Read the model definition and answer for the solid it produces. Units are mm, in the model's axes. Face numbers are marked on the shaded views. A direction names the side the tool comes from. Coordinates: 2 decimals unless noted, no trailing zeros. Order: outer loops, then holes, each group sorted by start corner. A loop starts at its lowest first (then second) coordinate and runs counter-clockwise, first axis right, second up. Notation, with made-up numbers: (-8.75, 72) -> (30.25, 72) arc R31 ccw to (30.25, 97) -> close; hole circle Ø6 at (-12.75, 50). An arc over 180 degrees is marked (long way). Return JSON: item names as keys, results as strings. Group by question number.
```python
from build123d import *

# Parameters (mm, degrees)
CASE_23X12P2X23_START                = -19
CASE_23X12P2X23_PROFILE_W            = 23
CASE_23X12P2X23_PROFILE_H            = 12.2
CASE_23X12P2X23_DEPTH                = 23
MOUNTING_EARS_33X12P2_START          = -2
MOUNTING_EARS_33X12P2_PROFILE_W      = 33
MOUNTING_EARS_33X12P2_PROFILE_H      = 12.2
MOUNTING_EARS_33X12P2_DEPTH          = 2
OUTPUT_ENVELOPE_NOT_SPLINE_START     = 4
OUTPUT_ENVELOPE_NOT_SPLINE_PROFILE_R = 2.5
OUTPUT_ENVELOPE_NOT_SPLINE_DEPTH     = 5
MOUNTING_HOLES_NOMINAL_START         = -50
MOUNTING_HOLES_NOMINAL_PROFILE_R     = 1.1
MOUNTING_HOLES_NOMINAL_DEPTH         = 80.702020133


with BuildPart() as part:
    # Case_23x12p2x23_profile → Case_23x12p2x23 (new body)
    with BuildSketch(Plane.XY.offset(CASE_23X12P2X23_START)):
        with Locations((5.5, 0)):
            Rectangle(CASE_23X12P2X23_PROFILE_W, CASE_23X12P2X23_PROFILE_H)
    extrude(amount=CASE_23X12P2X23_DEPTH)

    # Mounting_ears_33x12p2_profile → Mounting_ears_33x12p2 (add)
    with BuildSketch(Plane.XY.offset(MOUNTING_EARS_33X12P2_START)):
        with Locations((5.5, 0)):
            Rectangle(MOUNTING_EARS_33X12P2_PROFILE_W, MOUNTING_EARS_33X12P2_PROFILE_H)
    extrude(amount=MOUNTING_EARS_33X12P2_DEPTH)

    # Output_envelope_not_spline_profile → Output_envelope_not_spline (add)
    with BuildSketch(Plane.XY.offset(OUTPUT_ENVELOPE_NOT_SPLINE_START)):
        Circle(OUTPUT_ENVELOPE_NOT_SPLINE_PROFILE_R)
    extrude(amount=OUTPUT_ENVELOPE_NOT_SPLINE_DEPTH)

    # Mounting_holes_nominal_profile → Mounting_holes_nominal (cut, through all)
    with BuildSketch(Plane.XY.offset(MOUNTING_HOLES_NOMINAL_START)):
        with Locations(Location((-9, 0, 0), (0, 0, 180))):
            Circle(MOUNTING_HOLES_NOMINAL_PROFILE_R)
        with Locations(Location((20, 0, 0), (0, 0, 180))):
            Circle(MOUNTING_HOLES_NOMINAL_PROFILE_R)
    extrude(amount=MOUNTING_HOLES_NOMINAL_DEPTH, mode=Mode.SUBTRACT)


solid = part.part
```
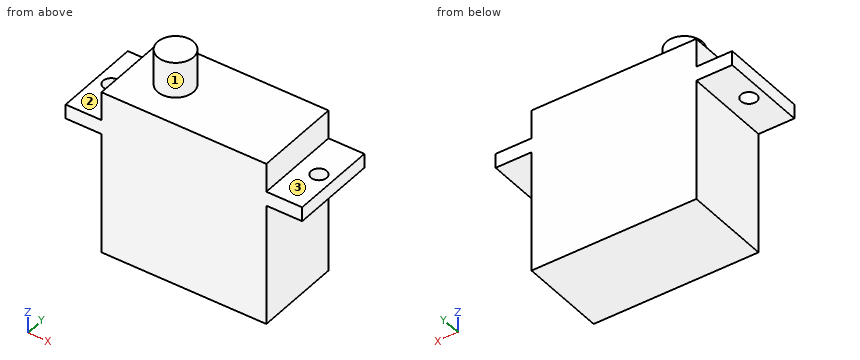
1. Straight lines are drawn through the part: L1, parallel to Y at x = -9, z = -1.4; L2, parallel to X at y = 2.75, z = -10.25; L3, parallel to Z at x = 20.5, y = -1.75. For each, find the intervals that lie inside material, in ascending order.
2. Find section A-A on x = -9. Determine the outline of the cut face in (y, z), and give its area (3 significant figures).
3. Find section D-D on y = 2. Determine the outline of the cut face in (x, z).
4. Find section C-C on x = 0. Determine the outline of the cut face in (y, z), and give its area (3 significant figures).
5. Given pin 1 (1.5 mm diameter, centred on y = -4, z = -9.5, fed in from +X); pin 2 (2 mm diameter, centred on y = -0.5, z = 3, fed in from -X); pin 3 (2.5 mm diameter, centred on x = -9.5, y = 1, fed in from -Z), each flat-ended and moving along its own axis, determine where each tip first touches the part or whether it passes through.
6. Find section B-B on y = 0. Determine the outline of the cut face in (x, z), and give its area (3 significant figures).
7. Which of the six approach directions +Z, -Z, +X, -X, +Y, -Y give full straight-line access (tool end or side, diameter ignored) to the marked faces 1, 2 and 3?
Result:
{
 "1": {"L1": "-6.1 to -1.1, 1.1 to 6.1", "L2": "-6 to 17", "L3": "-2 to 0"},
 "2": {"outline": "(-6.1, -2) -> (-1.1, -2) -> (-1.1, 0) -> (-6.1, 0) -> close; (1.1, -2) -> (6.1, -2) -> (6.1, 0) -> (1.1, 0) -> close", "area": "20.0 mm^2"},
 "3": {"outline": "(-11, -2) -> (-6, -2) -> (-6, -19) -> (17, -19) -> (17, -2) -> (22, -2) -> (22, 0) -> (17, 0) -> (17, 4) -> (1.5, 4) -> (1.5, 9) -> (-1.5, 9) -> (-1.5, 4) -> (-6, 4) -> (-6, 0) -> (-11, 0) -> close"},
 "4": {"outline": "(-6.1, -19) -> (6.1, -19) -> (6.1, 4) -> (2.5, 4) -> (2.5, 9) -> (-2.5, 9) -> (-2.5, 4) -> (-6.1, 4) -> close", "area": "306 mm^2"},
 "5": {"pin 1": "x = 17", "pin 2": "x = -6", "pin 3": "z = -2"},
 "6": {"outline": "(-11, -2) -> (-10.1, -2) -> (-10.1, 0) -> (-11, 0) -> close; (-7.9, -2) -> (-6, -2) -> (-6, -19) -> (17, -19) -> (17, -2) -> (18.9, -2) -> (18.9, 0) -> (17, 0) -> (17, 4) -> (2.5, 4) -> (2.5, 9) -> (-2.5, 9) -> (-2.5, 4) -> (-6, 4) -> (-6, 0) -> (-7.9, 0) -> close; (21.1, -2) -> (22, -2) -> (22, 0) -> (21.1, 0) -> close", "area": "565 mm^2"},
 "7": {"face 1": "+Z", "face 2": "+Z, -X, +Y, -Y", "face 3": "+Z, +X, +Y, -Y"}
}
